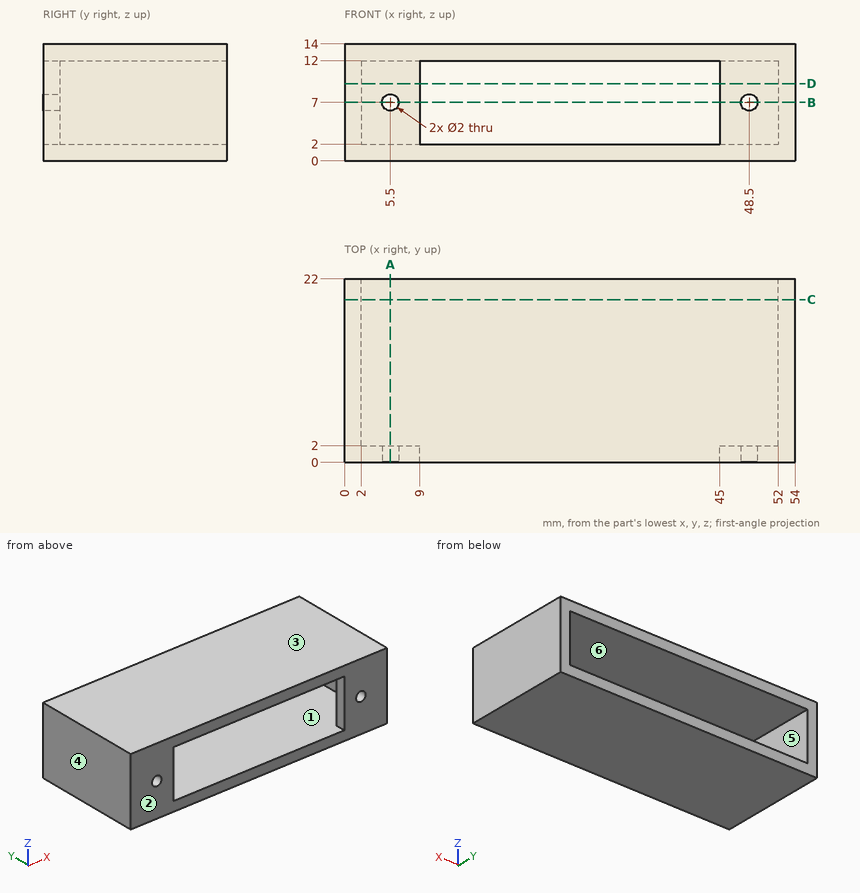
The drawing under review shows one solid part. Ordinate dimensions are in mm from its lowest x, y, z. A direction names the side the tool comes from. Give positions to 0.01 mm unless a question says otherwise; leave off trailing zeros. Order: outer loops, then holes, each group sorted by start corner. A loop starts at its lowest first (then second) coordinate and runs counter-clockwise, first axis right, second up. Notation, with made-up numbers: M 48.25,-9.75 L 76.25,-9.75 A22 ccw 76.25,0.25 Z; hole C 20.25,48 d11. An arc over 180 degrees is marked long. One line per question, with ' | ' between items. Start each with the question number.
Q1. We need section A-A (x = 5.5). Write out the cut boundary in (y, z).
Q2. We need section D-D (z = 9.25). Write out the cut boundary in (x, y), plus the area to 3 significant figures.
Q3. For L1, parallel to X at y = 0.8, z = 7; L2, parallel to Z at x = 26.5, y = 8.75; L3, parallel to X at y = 15, z = 5.75, list the stretches that pass through material, from the lowest coordinate up. Write a range as [from, to].
Q4. We need section B-B (z = 7). Write out the cut boundary in (x, y).
Q5. For pin 1 Ø6 at (x, z) = (14.5, 8.5) entering from +Y; pin 2 Ø4 at (y, z) = (19, 4) entering from -X; pin 3 Ø3.5 at (x, z) = (47.5, 5) entering from +Y, all flat-tipped, find the tip position at first contact; note any pin that passes through.
Q6. The part is to be moulded in two halves that separate along X. For the marked faces 3, 4, 5 and 6, say which applies: +X half, -X half, draft (parallel to the pull), parting line (faces both ways), or undercut.
Q7. We need section C-C (y = 19.5). Write out the cut boundary in (x, z).
Q8. Machinability: for the marked faces 1 and 2, which of the approach directions +Z, -Z, +X, -X, +Y, -Y give a long, thin tool a straight path to every point of the face, cutting with its end or side? Answer none if there is none.
Returned:
1) outline: M 0,0 L 22,0 L 22,2 L 2,2 L 2,6 L 0,6 Z; M 0,8 L 2,8 L 2,12 L 22,12 L 22,14 L 0,14 Z
2) outline: M 0,0 L 9,0 L 9,2 L 2,2 L 2,22 L 0,22 Z; M 45,0 L 54,0 L 54,22 L 52,22 L 52,2 L 45,2 Z | area: 116 mm2
3) L1: [0, 4.5], [6.5, 9], [45, 47.5], [49.5, 54] | L2: [0, 2], [12, 14] | L3: [0, 2], [52, 54]
4) outline: M 0,0 L 4.5,0 L 4.5,2 L 2,2 L 2,22 L 0,22 Z; M 6.5,0 L 9,0 L 9,2 L 6.5,2 Z; M 45,0 L 47.5,0 L 47.5,2 L 45,2 Z; M 49.5,0 L 54,0 L 54,22 L 52,22 L 52,2 L 49.5,2 Z
5) pin 1: through | pin 2: x = 0 | pin 3: y = 2
6) face 3: draft | face 4: -X half | face 5: undercut | face 6: undercut
7) outline: M 0,0 L 54,0 L 54,14 L 0,14 Z; hole M 2,2 L 52,2 L 52,12 L 2,12 Z
8) face 1: +Y | face 2: +Z, -Z, +X, -X, -Y
